Geometry: see drawing. Coordinates: mm, zero at the bounding-box minimum. Coordinates: 2 decimals unless noted, no trailing zeros. Loops run counter-clockwise (first coordinate to the right, second up) from the corner with the lowest first, then second, coordinate; pieces in that order, holes last.
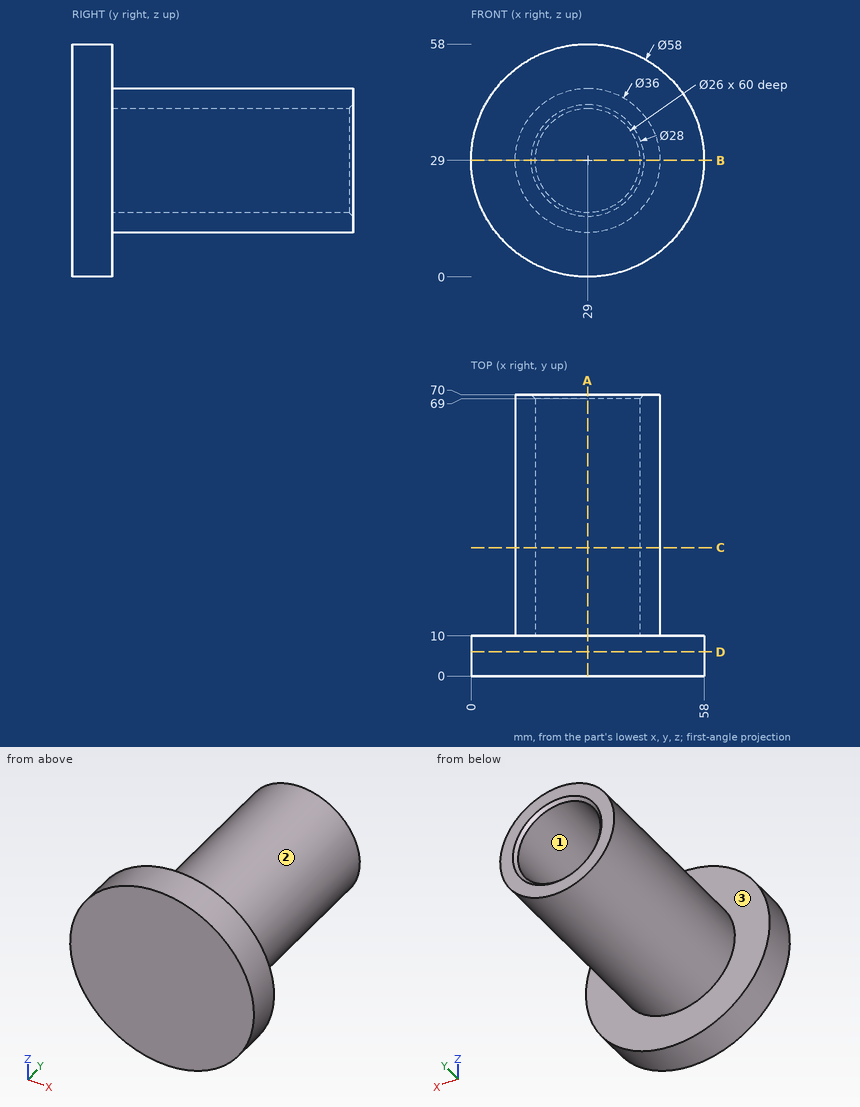
Item 1: Line query: L1, parallel to X at y = 24, z = 29; L2, parallel to Y at x = 4, z = 15; L3, parallel to X at y = 37.5, z = 27. Output: solid intervals per line, ascending.
Result:
L1: x = 11 to 16, 42 to 47
L2: y = 0 to 10
L3: x = 11.11 to 16.15, 41.85 to 46.89
Item 2: Contact query for flat-ended pins moving along their axis: P1, Ø1.5, axis at x = 43, y = 55, coming from the +Z side; P2, Ø1.5, axis at x = 31.5, y = 23, coming from the +Z side; P3, Ø10, axis at x = 49, y = 63, coming from the -Z side; P4, Ø1, axis at x = 46.5, z = 20, coming from the -Y side. Output: stop coordinate, or through.
Result:
P1: stops at z = 41.18
P2: stops at z = 46.91
P3: stops at z = 19.05
P4: stops at y = 0
Item 3: Section query C-C (y = 32). Output: boundary loops of the cut face in (x, z).
Result:
outline: circle Ø36 at (29, 29); hole circle Ø26 at (29, 29)
Item 4: Section query D-D (y = 6). Output: boundary loops of the cut face in (x, z), then the cut area to 3 significant figures.
Result:
outline: circle Ø58 at (29, 29)
area: 2,640 mm2
Item 5: Section query B-B (z = 29). Output: boundary loops of the cut face in (x, y), then the cut area to 3 significant figures.
Result:
outline: (0, 0) - (58, 0) - (58, 10) - (47, 10) - (47, 70) - (43, 70) - (42, 69) - (42, 10) - (16, 10) - (16, 69) - (15, 70) - (11, 70) - (11, 10) - (0, 10) - close
area: 1,180 mm2
Item 6: Section query A-A (x = 29). Output: boundary loops of the cut face in (y, z), then the cut area to 3 significant figures.
Result:
outline: (0, 0) - (10, 0) - (10, 11) - (70, 11) - (70, 15) - (69, 16) - (10, 16) - (10, 42) - (69, 42) - (70, 43) - (70, 47) - (10, 47) - (10, 58) - (0, 58) - close
area: 1,180 mm2
Item 7: Mould query, pull axis Z, two halves, no side actions, for the marked faces 1, 2 and 3. Classes: +Z half, -Z half, draft (parallel to the pull), parting line (faces both ways), or undercut.
Result:
face 1: undercut
face 2: parting line
face 3: draft
